Can you work these out from the model? Positions are in its coordinate system, mm. Round coordinates to 2 decimals unless told otherwise and drop trailing zeros. Write item = value, one per line.
from build123d import *

# Parameters (mm, degrees)
SKETCH_W        = 20
SKETCH_H        = 20
PAD_DEPTH       = 400
SKETCH001_R     = 2.5
POCKET_DEPTH    = 400.001
POCKET001_DEPTH = 400.001


with BuildPart() as part:
    # Sketch → Pad (new body)
    with BuildSketch(Plane.XY):
        Rectangle(SKETCH_W, SKETCH_H)
    extrude(amount=PAD_DEPTH)

    # Sketch001 (on Face6 of Pad) → Pocket (cut, through all)
    with BuildSketch(Plane.XY.offset(400)):
        Circle(SKETCH001_R)
        Polygon((-3.1, 10), (3.1, 10), (3.1, 8), (6.232233, 8), (2.132233, 3.9), (-2.132233, 3.9), (-6.232233, 8), (-3.1, 8), align=None)
        Polygon((-3.1, -8), (-6.232233, -8), (-2.132233, -3.9), (2.132233, -3.9), (6.232233, -8), (3.1, -8), (3.1, -10), (-3.1, -10), align=None)
    extrude(amount=-POCKET_DEPTH, mode=Mode.SUBTRACT)

    # Sketch002 (on Face2 of Pocket) → Pocket001 (cut, through all)
    with BuildSketch(Plane(origin=(0, 0, 0), x_dir=(1, 0, 0), z_dir=(0, 0, -1))):
        Polygon((-10, -3.1), (-8, -3.1), (-8, -6.232233), (-3.9, -2.132233), (-3.9, 2.132233), (-8, 6.232233), (-8, 3.1), (-10, 3.1), align=None)
        Polygon((3.9, -2.132233), (3.9, 2.132233), (8, 6.232233), (8, 3.1), (10, 3.1), (10, -3.1), (8, -3.1), (8, -6.232233), align=None)
    extrude(amount=-POCKET001_DEPTH, mode=Mode.SUBTRACT)


solid = part.part
1. I'm going to push flat-ended pins straight in: pin 1 (2 mm diameter, centred on x = -0.5, z = 195, fed in from -Y); pin 2 (4.5 mm diameter, centred on x = 0, y = 0, fed in from +Z); pin 3 (1.3 mm diameter, centred on x = 0, z = 234, fed in from +Y). Where does each tip first touch, or does it pass through?
Entries:
pin_1 = -3.9
pin_2 = through
pin_3 = 3.9
2. I need wall thicknesses on line 1 (Y direction, x = 0, z = 155.5); line 2 (Y direction, x = -9, z = 306). Which ranges of each line are inside material? Lowest first, please. Write a range as [from, to].
Entries:
line_1 = [-3.9, -2.5], [2.5, 3.9]
line_2 = [-10, -3.1], [3.1, 10]
3. We'd pull the mould along Z, two halves only. Please class faces 1 (the flat face through (7, -10, 197)), 2 (the flat face through (2, 2, 400)), 3 (the flat face through (2, 2, 0)): released by +Z, released by -Z, zero draft, split by the parting line, or undercut.
Entries:
face_1 = zero draft
face_2 = released by +Z
face_3 = released by -Z
